Geometry check sheet. Reference: the model listing, model coordinates, mm. A direction names the side the tool comes from. Round coordinates to 2 decimals unless told otherwise and drop trailing zeros. Write each loop counter-clockwise with the first axis right and the second up, starting at its lowest first coordinate (ties: lowest second). Pieces come first, ordered by that corner, then holes. Notation, with made-up numbers: (-12.75, 60.25) -> (-7.75, 60.25) arc R21 cw to (-7.75, 94.25) -> close; hole circle Ø6 at (24, 50.5). An arc over 180 degrees is marked (long way). Put each result on its own line as item: value. Start each with the question number.
from build123d import *

# Parameters (mm, degrees)
SKETCH1_R           = 2.5
BOSS_EXTRUDE1_DEPTH = 10
BOSS_EXTRUDE2_DEPTH = 120
SKETCH3_R           = 100
SKETCH3_R_2         = 10
BOSS_EXTRUDE3_DEPTH = 5


with BuildPart() as part:
    # Sketch1 → Boss-Extrude1 (new body)
    with BuildSketch(Plane.XY):
        with BuildLine():
            Line((10, 99.498743711), (10, 104.292304576))
            Line((10, 104.292304576), (4, 115))
            Line((4, 115), (-4, 115))
            Line((-4, 115), (-10, 104.292304576))
            Line((-10, 104.292304576), (-10, 99.498743711))
            ThreePointArc((-10, 99.498743711), (-70.710678119, 70.710678119), (-99.498743711, 10))
            Line((-99.498743711, 10), (-104.292304576, 10))
            Line((-104.292304576, 10), (-115, 4))
            Line((-115, 4), (-115, -4))
            Line((-115, -4), (-104.292304576, -10))
            Line((-104.292304576, -10), (-99.498743711, -10))
            ThreePointArc((-99.498743711, -10), (-70.710678119, -70.710678119), (-10, -99.498743711))
            Line((-10, -99.498743711), (-10, -104.292304576))
            Line((-10, -104.292304576), (-4, -115))
            Line((-4, -115), (4, -115))
            Line((4, -115), (10, -104.292304576))
            Line((10, -104.292304576), (10, -99.498743711))
            ThreePointArc((10, -99.498743711), (70.710678119, -70.710678119), (99.498743711, -10))
            Line((99.498743711, -10), (104.292304576, -10))
            Line((104.292304576, -10), (115, -4))
            Line((115, -4), (115, 4))
            Line((115, 4), (104.292304576, 10))
            Line((104.292304576, 10), (99.498743711, 10))
            ThreePointArc((99.498743711, 10), (70.710678119, 70.710678119), (10, 99.498743711))
        make_face()
        with Locations((-106.562672681, 0)):
            Circle(SKETCH1_R, mode=Mode.SUBTRACT)
        with Locations((106.562672681, 0)):
            Circle(SKETCH1_R, mode=Mode.SUBTRACT)
        with Locations((0, 106.562672681)):
            Circle(SKETCH1_R, mode=Mode.SUBTRACT)
        with Locations((0, -106.562672681)):
            Circle(SKETCH1_R, mode=Mode.SUBTRACT)
    extrude(amount=BOSS_EXTRUDE1_DEPTH)

    # Sketch2 → Boss-Extrude2 (add)
    with BuildSketch(Plane.XY.offset(10)):
        Polygon((-61.183161588, -50.705696973), (-65.740333213, -45.487250194), (-72.538226504, -46.824653202), (-74.77894817, -53.380502987), (-70.221776545, -58.598949766), (-63.423883254, -57.261546759), align=None)
        Polygon((34.031190696, -84.892949499), (34.859909403, -78.01448853), (29.317346819, -73.857566592), (22.946065527, -76.579105623), (22.117346819, -83.457566592), (27.659909403, -87.61448853), align=None)
        Polygon((-67.13062022, 42.519722439), (-63.575825884, 48.466438948), (-66.948436282, 54.518339402), (-73.875841015, 54.623523347), (-77.430635351, 48.676806839), (-74.058024953, 42.624906385), align=None)
        Polygon((19.694156606, 76.984330633), (26.448311953, 75.441156778), (31.161817388, 80.518839962), (29.121167475, 87.139697001), (22.367012128, 88.682870856), (17.653506693, 83.605187672), align=None)
        Polygon((79.302278382, 5.059210493), (79.921781616, -1.841239909), (86.207498579, -4.75495957), (91.873712307, -0.768228831), (91.254209072, 6.13222157), (84.96849211, 9.045941232), align=None)
    extrude(amount=BOSS_EXTRUDE2_DEPTH)

    # Sketch3 → Boss-Extrude3 (add)
    with BuildSketch(Plane.XY.offset(130)):
        Circle(SKETCH3_R)
        Circle(SKETCH3_R_2, mode=Mode.SUBTRACT)
    extrude(amount=BOSS_EXTRUDE3_DEPTH)


solid = part.part
(1) Sectioned sample at A-A (z = 96). State how many separate pieces and enclosed holes the cut face has, and give its area (3 significant figures).
(2) Set-up check for faces 5 (the flat face through (-73.643, -50.057, 69.16)), 6 (the flat face through (79.608, 1.657, 69.16)), 7 (the flat face through (34.44, -81.5, 69.16)): record each of +Z, -Z, +X, -X, +Y, -Y from which the full face is reachable in a straight line by a thin tool's end or side.
(3) Sectioned sample at C-C (x = -91.5). Record the cut outline in (y, z), and give its area (3 significant figures).
(4) Sectioned sample at B-B (x = -19.5). Record the cut outline in (y, z).
(5) Mould release check, pull along Z, two halves, no side actions. Record for faces 1 (the flat face through (-2, 2, 10)), 2 (the flat face through (-115, 0, 5)), 3 (the flat face through (22.538, -79.97, 69.16)), 4 (the flat face through (-1, -21, 135)): +Z half, -Z half, draft (parallel to the pull), parting line (faces both ways), or undercut.
(6) Go/stop test with flat-tipped pins: pin 1 Ø2.5 at (x, z) = (-102, 3) entering from -Y; pin 2 Ø1.4 at (y, z) = (-102.5, 6.5) entering from -X; pin 3 Ø4 at (x, z) = (-103, 7) entering from +Y. Record where each tip stops, or that it passes through.
(7) Material ranges on L1, parallel to Y at x = 0, z = 7; L2, parallel to Z at x = 56.5, y = -15.5; L3, parallel to Y at x = -64, z = 18, recorded low to high. Write a range as from..to.
Found:
1. separate pieces: 5
1. enclosed holes: 0
1. area: 624 mm2
2. face 5: -X
2. face 6: -X, -Y
2. face 7: +X, -Y
3. outline: (-40.35, 0) -> (40.35, 0) -> (40.35, 10) -> (-40.35, 10) -> close; (-40.35, 130) -> (40.35, 130) -> (40.35, 135) -> (-40.35, 135) -> close
3. area: 1,210 mm2
4. outline: (-98.08, 0) -> (98.08, 0) -> (98.08, 10) -> (-98.08, 10) -> close; (-98.08, 130) -> (98.08, 130) -> (98.08, 135) -> (-98.08, 135) -> close
5. face 1: undercut
5. face 2: draft
5. face 3: undercut
5. face 4: +Z half
6. pin 1: y = -10
6. pin 2: x = -10
6. pin 3: y = 10
7. L1: -115..-109.06, -104.06..104.06, 109.06..115
7. L2: 0..10, 130..135
7. L3: -57.37..-47.48, 47.76..49.23
